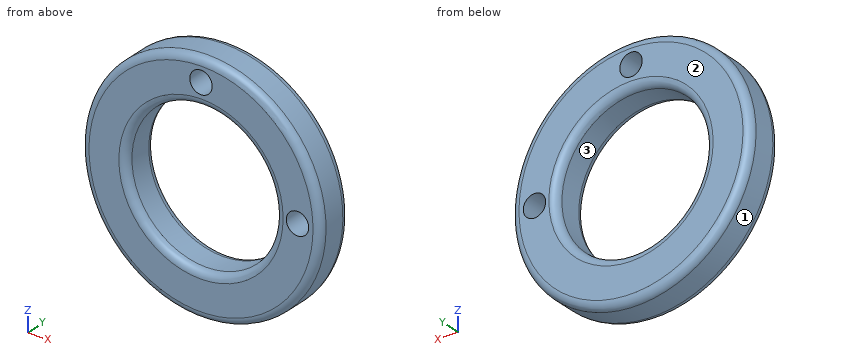
```python
from build123d import *

# Parameters (mm, degrees)
SKETCH1_R           = 16
SKETCH1_R_2         = 10
SKETCH1_R_3         = 1.5
BOSS_EXTRUDE1_DEPTH = 5
FILLET1_R           = 1


with BuildPart() as part:
    # Sketch1 → Boss-Extrude1 (new body)
    with BuildSketch(Plane(origin=(0, 0, 0), x_dir=(1, 0, 0), z_dir=(0, 1, 0))):
        with Locations(Location((0, 0, 0), (0, 0, 270))):
            Circle(SKETCH1_R)
        with Locations(Location((0, 0, 0), (0, 0, 270))):
            Circle(SKETCH1_R_2, mode=Mode.SUBTRACT)
        with Locations(Location((0, -13, 0), (0, 0, 270))):
            Circle(SKETCH1_R_3, mode=Mode.SUBTRACT)
        with Locations(Location((12.925776556, 0, 0), (0, 0, 270))):
            Circle(SKETCH1_R_3, mode=Mode.SUBTRACT)
    extrude(amount=BOSS_EXTRUDE1_DEPTH)

    # Fillet1
    fillet1_edges = [part.edges().sort_by_distance(p)[0] for p in [
        (0, 0, -16),
        (0, 5, -16),
        (0, 0, -10),
        (0, 5, -10),
    ]]
    fillet(fillet1_edges, radius=FILLET1_R)


solid = part.part
```
Here's how the part is built. I have some questions about the finished solid (model axes, mm). Face numbers are marked on the shaded views. Give positions to 0.01 mm unless a question says otherwise; leave off trailing zeros. Order: outer loops, then holes, each group sorted by start corner. A loop starts at its lowest first (then second) coordinate and runs counter-clockwise, first axis right, second up. Notation, with made-up numbers: M 72,46.25 L 94,46.25 A21 ccw 94,50.25 Z; hole C -1.75,44 d10. An arc over 180 degrees is marked long. Use a Markdown table: item, result. Add a question column.
1. Suppose I cut it at C-C (y = 2.05). List the corners of the cut face in (x, z) for me.
2. Suppose I cut it at A-A (x = 0). List the corners of the cut face in (y, z) for me, and give its area (3 significant figures).
3. For pin 1 Ø1 at (y, z) = (1.5, -5) entering from -X; pin 2 Ø3 at (y, z) = (1, 10.5) entering from -X, each with a flat end and sliding along its axis, tell me the tip position at first contact or that it passes through.
4. Suppose I cut it at B-B (z = 0). List the corners of the cut face in (x, y) for me.
5. If we mould it in two halves opening along Z, with no side actions, what happens to the marked faces 1, 2 and 3? For each: +Z half, -Z half, draft (parallel to the pull), parting line (faces both ways), or undercut.
6. Suppose I cut it at D-D (y = 4.6). List the corners of the cut face in (x, z) for me.
7. I need wall thicknesses on probe 1 along X at (y, z) = (1.7, 0); probe 2 along Z at (x, y) = (-0.5, 2.95); probe 3 along X at (y, z) = (3.8, 13). Which ranges of each line are inside material? Lowest first, please. Write a range as from..to.
Results list:
| question | item | result |
|---|---|---|
| 1 | outline | C 0,0 d32; hole C 0,0 d20; hole C 0,13 d3; hole C 12.93,0 d3 |
| 2 | outline | M 0,-15 A1 ccw 1,-16 L 4,-16 A1 ccw 5,-15 L 5,-11 A1 ccw 4,-10 L 1,-10 A1 ccw 0,-11 Z; M 0,11 A1 ccw 1,10 L 4,10 A1 ccw 5,11 L 5,11.5 L 0,11.5 Z; M 0,14.5 L 5,14.5 L 5,15 A1 ccw 4,16 L 1,16 A1 ccw 0,15 Z |
| 2 | area | 43.3 mm² |
| 3 | pin 1 | stops at x = -15.35 |
| 3 | pin 2 | stops at x = -13.23 |
| 4 | outline | M -16,1 A1 ccw -15,0 L -11,0 A1 ccw -10,1 L -10,4 A1 ccw -11,5 L -15,5 A1 ccw -16,4 Z; M 10,1 A1 ccw 11,0 L 11.43,0 L 11.43,5 L 11,5 A1 ccw 10,4 Z; M 14.43,0 L 15,0 A1 ccw 16,1 L 16,4 A1 ccw 15,5 L 14.43,5 Z |
| 5 | face 1 | parting line |
| 5 | face 2 | draft |
| 5 | face 3 | undercut |
| 6 | outline | C 0,0 d31.6; hole C 0,0 d20.4; hole C 0,13 d3; hole C 12.93,0 d3 |
| 7 | probe 1 | x = -16..-10, 10..11.43, 14.43..16 |
| 7 | probe 2 | z = -15.99..-9.99, 9.99..11.59, 14.41..15.99 |
| 7 | probe 3 | x = -9.33..-1.5, 1.5..9.33 |
